Source: CAD feature listing. Evaluate the final solid. Frame: model axes, mm. A direction names the side the tool comes from. Give positions to 0.01 mm unless a question says otherwise; leave off trailing zeros. Loops run counter-clockwise (first coordinate to the right, second up) from the corner with the lowest first, then second, coordinate; pieces in that order, holes last. Notation, with made-up numbers: (-23, -11.75) -> (-8, -11.75) arc R17 cw to (-8, 20.25) -> close; hole circle Ø9 at (-37.75, 70). An arc over 180 degrees is marked (long way). Return JSON: item names as keys, results as strings. Group by question number.
(1) Cut plane D-D on z = -7. Return loops of the section in (x, y), then the cut area to 3 significant figures.
(2) Cut plane B-B on x = 0. Return loops of the section in (y, z), then the cut area to 3 significant figures.
(3) Draft query along Z for faces 4 (the face through (-10, 4, 0)), 5 (the face through (-3.32, 5.13, 0.74)), 6 (the face through (0, 5, -10)). Return one class per face: released by +Z, released by -Z, zero draft, split by the parting line, or undercut.
(4) Ray query, line 1 (X direction, y = 4, z = 0); line 2 (X direction, y = 7.5, z = 0); line 3 (X direction, y = 6.75, z = 4). Return the intervals inside material, ascending. Write a range as from..to.
(5) Cut plane C-C on y = 6.25. Return loops of the section in (x, z), then the cut area to 3 significant figures.
(6) Cut plane A-A on z = 3. Return loops of the section in (x, y), then the cut area to 3 significant figures.
(7) Access query for faces 1 (the face through (5.2, 8, 0)), 2 (the face through (10, 4, 0)), 3 (the face through (-5.2, 8, 0)). Directions: +Z, -Z, +X, -X, +Y, -Y. A direction counts if a zero-diameter tool reaches every point of the face in a straight line with its end or side. Return the directions, or none.
(8) Pin query (flat end, axial travel): pin 1 (3 mm diameter, centred on x = -8, z = -2.5, fed in from +Y); pin 2 (1.2 mm diameter, centred on y = 7.5, z = -3.5, fed in from -X); pin 3 (3 mm diameter, centred on y = 7.5, z = 1, fed in from +X). Return the tip coordinate at first contact, or that it passes through.
```python
from build123d import *

# Parameters (mm, degrees)
EXTRUDE_1_DEPTH        = 10
HOLE_WIZARD_M8_1_D     = 6.8
HOLE_WIZARD_M8_1_DEPTH = 19.75
HOLE_WIZARD_M8_1_TIP   = 2.042926105


with BuildPart() as part:
    # 草图1 → 凸台-拉伸1 (new, symmetric)
    with BuildSketch(Plane.XY):
        with BuildLine():
            Line((-5, 0), (5, 0))
            ThreePointArc((5, 0), (7.707230765, 1.475471539), (10, 3.53686037))
            Line((10, 3.53686037), (10, 4.9))
            ThreePointArc((10, 4.9), (9.853553391, 5.253553391), (9.5, 5.4))
            Line((9.5, 5.4), (5.7, 5.4))
            ThreePointArc((5.7, 5.4), (5.346446609, 5.546446609), (5.2, 5.9))
            Line((5.2, 5.9), (5.2, 9.9))
            ThreePointArc((5.2, 9.9), (5.053553391, 10.253553391), (4.7, 10.4))
            Line((4.7, 10.4), (-4.7, 10.4))
            ThreePointArc((-4.7, 10.4), (-5.053553391, 10.253553391), (-5.2, 9.9))
            Line((-5.2, 9.9), (-5.2, 5.9))
            ThreePointArc((-5.2, 5.9), (-5.346446609, 5.546446609), (-5.7, 5.4))
            Line((-5.7, 5.4), (-9.5, 5.4))
            ThreePointArc((-9.5, 5.4), (-9.853553391, 5.253553391), (-10, 4.9))
            Line((-10, 4.9), (-10, 3.53686037))
            ThreePointArc((-10, 3.53686037), (-7.707230765, 1.475471539), (-5, 0))
        make_face()
    extrude(amount=EXTRUDE_1_DEPTH, both=True)

    # M8 螺纹孔1
    with Locations(Plane.ZX.offset(10.4)):
        with Locations((0, 0)):
            Hole(HOLE_WIZARD_M8_1_D / 2, depth=HOLE_WIZARD_M8_1_DEPTH)
            with Locations((0, 0, -(HOLE_WIZARD_M8_1_DEPTH + HOLE_WIZARD_M8_1_TIP / 2))):  # 118° drill point
                Cone(0, HOLE_WIZARD_M8_1_D / 2, HOLE_WIZARD_M8_1_TIP, mode=Mode.SUBTRACT)


solid = part.part
```
Answers:
{
 "1": {"outline": "(-10, 3.54) arc R13.25 ccw to (-5, 0) -> (5, 0) arc R13.25 ccw to (10, 3.54) -> (10, 4.9) arc R0.5 ccw to (9.5, 5.4) -> (5.7, 5.4) arc R0.5 cw to (5.2, 5.9) -> (5.2, 9.9) arc R0.5 ccw to (4.7, 10.4) -> (-4.7, 10.4) arc R0.5 ccw to (-5.2, 9.9) -> (-5.2, 5.9) arc R0.5 cw to (-5.7, 5.4) -> (-9.5, 5.4) arc R0.5 ccw to (-10, 4.9) -> close", "area": "145 mm²"},
 "2": {"outline": "(0, -10) -> (10.4, -10) -> (10.4, -3.4) -> (0, -3.4) -> close; (0, 3.4) -> (10.4, 3.4) -> (10.4, 10) -> (0, 10) -> close", "area": "137 mm²"},
 "3": {"face 4": "zero draft", "face 5": "undercut", "face 6": "released by -Z"},
 "4": {"line 1": "-10..-3.4, 3.4..10", "line 2": "-5.2..-3.4, 3.4..5.2", "line 3": "-5.2..5.2"},
 "5": {"outline": "(-5.2, -10) -> (5.2, -10) -> (5.2, 10) -> (-5.2, 10) -> close; hole circle Ø6.8 at (0, 0)", "area": "172 mm²"},
 "6": {"outline": "(-10, 3.54) arc R13.25 ccw to (-5, 0) -> (-1.6, 0) -> (-1.6, 10.4) -> (-4.7, 10.4) arc R0.5 ccw to (-5.2, 9.9) -> (-5.2, 5.9) arc R0.5 cw to (-5.7, 5.4) -> (-9.5, 5.4) arc R0.5 ccw to (-10, 4.9) -> close; (1.6, 0) -> (5, 0) arc R13.25 ccw to (10, 3.54) -> (10, 4.9) arc R0.5 ccw to (9.5, 5.4) -> (5.7, 5.4) arc R0.5 cw to (5.2, 5.9) -> (5.2, 9.9) arc R0.5 ccw to (4.7, 10.4) -> (1.6, 10.4) -> close", "area": "112 mm²"},
 "7": {"face 1": "+Z, -Z, +X, +Y", "face 2": "+Z, -Z, +X, +Y, -Y", "face 3": "+Z, -Z, -X, +Y"},
 "8": {"pin 1": "y = 5.4", "pin 2": "x = -5.2", "pin 3": "x = 5.2"}
}
